from build123d import *

# Parameters (mm, degrees)
F2_DEPTH     = 1.524
F3_DEPTH     = 0.762
F4_T1_DEPTH  = 21.59
F4_T3_DEPTH  = 15.24
F4_T6_ANGLE  = 90
F4_T8_ANGLE  = 90
F4_T10_ANGLE = 90
F4_T12_ANGLE = 90


# Not quite as in the source:
# - a fillet or chamfer that OpenCascade refuses, or shapes differently, is made with other operations: its cross-section is extruded or revolved along the edge and cut away or added


with BuildPart() as f2:
    # F1 (on face) → F2 (new body)
    with BuildSketch(Plane.XY):
        with BuildLine():
            ThreePointArc((-45.0744511747, 18.5649100114), (-44.144515205, 16.3198459811), (-41.8994511747, 15.3899100114))
            Line((-41.8994511747, 15.3899100114), (-33.8222511747, 15.3899100114))
            ThreePointArc((-33.8222511747, 15.3899100114), (-31.5771871445, 16.3198459811), (-30.6472511747, 18.5649100114))
            Line((-30.6472511747, 18.5649100114), (-30.6472511747, 33.5509100114))
            ThreePointArc((-30.6472511747, 33.5509100114), (-31.5771871445, 35.7959740417), (-33.8222511747, 36.7259100114))
            Line((-33.8222511747, 36.7259100114), (-41.8994511747, 36.7259100114))
            ThreePointArc((-41.8994511747, 36.7259100114), (-44.144515205, 35.7959740417), (-45.0744511747, 33.5509100114))
            Line((-45.0744511747, 33.5509100114), (-45.0744511747, 18.5649100114))
        make_face()
    extrude(amount=F2_DEPTH)

    # F0 (on Top) → F3 (join)
    with BuildSketch(Plane.XY):
        with BuildLine():
            ThreePointArc((-48.6558511747, 15.2629100114), (-47.725915205, 13.0178459811), (-45.4808511747, 12.0879100114))
            Line((-45.4808511747, 12.0879100114), (-30.2408511747, 12.0879100114))
            ThreePointArc((-30.2408511747, 12.0879100114), (-27.9957871445, 13.0178459811), (-27.0658511747, 15.2629100114))
            Line((-27.0658511747, 15.2629100114), (-27.0658511747, 36.8529100114))
            ThreePointArc((-27.0658511747, 36.8529100114), (-27.9957871445, 39.0979740417), (-30.2408511747, 40.0279100114))
            Line((-30.2408511747, 40.0279100114), (-45.4808511747, 40.0279100114))
            ThreePointArc((-45.4808511747, 40.0279100114), (-47.725915205, 39.0979740417), (-48.6558511747, 36.8529100114))
            Line((-48.6558511747, 36.8529100114), (-48.6558511747, 15.2629100114))
        make_face()
    extrude(amount=-F3_DEPTH)

    # F4: chamfer of 2.54 x 1.4664696837 on 8 edges, made by hand

    # F4_s2 → F4_t1 (cut)
    with BuildSketch(Plane.XZ.offset(-36.8529100114)):
        Polygon((-48.6558511747, 0.7044696837), (-46.1158511747, -0.762), (-48.6558511747, -0.762), align=None)
        Polygon((-29.6058511747, -0.762), (-27.0658511747, 0.7044696837), (-27.0658511747, -0.762), align=None)
    extrude(amount=F4_T1_DEPTH, mode=Mode.SUBTRACT)

    # F4_s4 → F4_t3 (cut)
    with BuildSketch(Plane.YZ.offset(-45.4808511747)):
        Polygon((37.4879100114, -0.762), (40.0279100114, 0.7044696837), (40.0279100114, -0.762), align=None)
        Polygon((12.0879100114, 0.7044696837), (14.6279100114, -0.762), (12.0879100114, -0.762), align=None)
    extrude(amount=F4_T3_DEPTH, mode=Mode.SUBTRACT)

    # F4_s5 → F4_t6 (revolve, cut)
    with BuildSketch(Plane.YZ.offset(-45.4808511747)):
        Polygon((37.4879100114, -0.762), (40.0279100114, 0.7044696837), (40.0279100114, -0.762), align=None)
    revolve(axis=Axis((-45.4808511747, 36.8529100114, -0.762), (0, 0, 1)), revolution_arc=F4_T6_ANGLE, mode=Mode.SUBTRACT)

    # F4_s7 → F4_t8 (revolve, cut)
    with BuildSketch(Plane.XZ.offset(-36.8529100114)):
        Polygon((-29.6058511747, -0.762), (-27.0658511747, 0.7044696837), (-27.0658511747, -0.762), align=None)
    revolve(axis=Axis((-30.2408511747, 36.8529100114, -0.762), (0, 0, 1)), revolution_arc=F4_T8_ANGLE, mode=Mode.SUBTRACT)

    # F4_s9 → F4_t10 (revolve, cut)
    with BuildSketch(Plane.YZ.offset(-30.2408511747)):
        Polygon((14.6279100114, -0.762), (12.0879100114, 0.7044696837), (12.0879100114, -0.762), align=None)
    revolve(axis=Axis((-30.2408511747, 15.2629100114, -0.762), (0, 0, 1)), revolution_arc=F4_T10_ANGLE, mode=Mode.SUBTRACT)

    # F4_s11 → F4_t12 (revolve, cut)
    with BuildSketch(Plane.XZ.offset(-15.2629100114)):
        Polygon((-48.6558511747, 0.7044696837), (-46.1158511747, -0.762), (-48.6558511747, -0.762), align=None)
    revolve(axis=Axis((-45.4808511747, 15.2629100114, -0.762), (0, 0, 1)), revolution_arc=F4_T12_ANGLE, mode=Mode.SUBTRACT)


solid = f2.part
Design review of the part built by this model. Coordinates are the model's own, in mm. A direction names the side the tool comes from. Round coordinates to 2 decimals unless told otherwise and drop trailing zeros. Order: outer loops, then holes, each group sorted by start corner. A loop starts at its lowest first (then second) coordinate and runs counter-clockwise, first axis right, second up.
1) Consider section A-A (z = 0.65). State the section outline as (x, y) points (3 decimals).
The answers:
outline: (-45.074, 18.565) arc R3.175 ccw to (-41.899, 15.39) - (-33.822, 15.39) arc R3.175 ccw to (-30.647, 18.565) - (-30.647, 33.551) arc R3.175 ccw to (-33.822, 36.726) - (-41.899, 36.726) arc R3.175 ccw to (-45.074, 33.551) - close
2) Consider section B-B (y = 27). State the section outline as (x, z) points.
The answers:
outline: (-47.44, 0) - (-46.12, -0.76) - (-29.61, -0.76) - (-28.29, 0) - (-30.65, 0) - (-30.65, 1.52) - (-45.07, 1.52) - (-45.07, 0) - close
3) Machinability: for faces 4 (the cylindrical face through (-31.55, 35.77, 0.75)), 5 (the flat face through (-38, 15.39, 1)), 6 (the flat face through (-47, 26, 0)), which of the approach directions +Z, -Z, +X, -X, +Y, -Y give a long, thin tool a straight path to every point of the face, cutting with its end or side? Answer none if there is none.
The answers:
face 4: +Z, +X, +Y
face 5: +Z, +X, -X, -Y
face 6: +Z
4) Draft analysis for pull direction Z (two halves, no side actions). For faces 1 (the flat face through (-28.96, 26.21, -0.39)), 2 (the flat face through (-38, 26, 1.524)), 3 (the flat face through (-30.647, 26, 1)), state which applies: released by +Z, released by -Z, zero draft, split by the parting line, or undercut.
The answers:
face 1: released by -Z
face 2: released by +Z
face 3: zero draft
5) For L1, parallel to X at y = 20, z = 1.35; L2, parallel to Y at x = -39, z = 1.2; L3, parallel to Z at x = -30.25, y = 18.75, list the stretches that pass through material, from the lowest coordinate up.
The answers:
L1: x = -45.07 to -30.65
L2: y = 15.39 to 36.73
L3: z = -0.76 to 0
6) Clearance check with flat-ended pins moving along their axes: pin 1 Ø1.2 at (y, z) = (22.5, 1) entering from -X; pin 2 Ø0.8 at (x, z) = (-38, 1) entering from +Y; pin 3 Ø0.5 at (y, z) = (26, 1) entering from +X. State where each tip first meets the part, or that it passes through.
The answers:
pin 1: stops at x = -45.07
pin 2: stops at y = 36.73
pin 3: stops at x = -30.65
